Could you check a few things on this drawing? It's one solid part, dimensions in mm from its lowest x, y, z. A direction names the side the tool comes from. Give positions to 0.01 mm unless a question says otherwise; leave off trailing zeros. Loops run counter-clockwise (first coordinate to the right, second up) from the corner with the lowest first, then second, coordinate; pieces in that order, holes last. Notation, with made-up numbers: (85.25, 39.5) - (111.25, 39.5) arc R29 ccw to (111.25, 60.5) - close; hole circle Ø2 at (54, -22.75). An arc over 180 degrees is marked (long way). Return JSON: item names as keys, results as strings. Group by question number.
(1) If we mould it in two halves opening along X, with no side actions, what happens to the marked faces 3, 4, 5 and 6? For each: released by +X, released by -X, zero draft, split by the parting line, or undercut.
(2) I need wall thicknesses on probe 1 along X at (y, z) = (2.95, 6.5); probe 2 along Y at (x, z) = (10.25, 7.25). Which ranges of each line are inside material? Lowest first, please. Write a range as [from, to].
(3) For P1, Ø4.5, axis at x = 6, z = 5.5, coming from the +Y side; P2, Ø1.5, axis at x = 2.5, y = 0.5, coming from the +Z side, each with a flat end and sliding along its axis, tell me the tip position at first contact or that it passes through.
(4) If we section it at B-B (y = 4.75): Please give me the cut outline in (x, z), then the cut area to 3 significant figures.
(5) On a 3-axis mill with a long thin cutter (end or side, diameter ignored), from which of +Z, -Z, +X, -X, +Y, -Y can I reach the whole of each face in a straight line? I mean the marked faces 1 and 2. Say none if no direction works.
(6) If we section it at A-A (z = 6.5): Please give me the cut outline in (x, y).
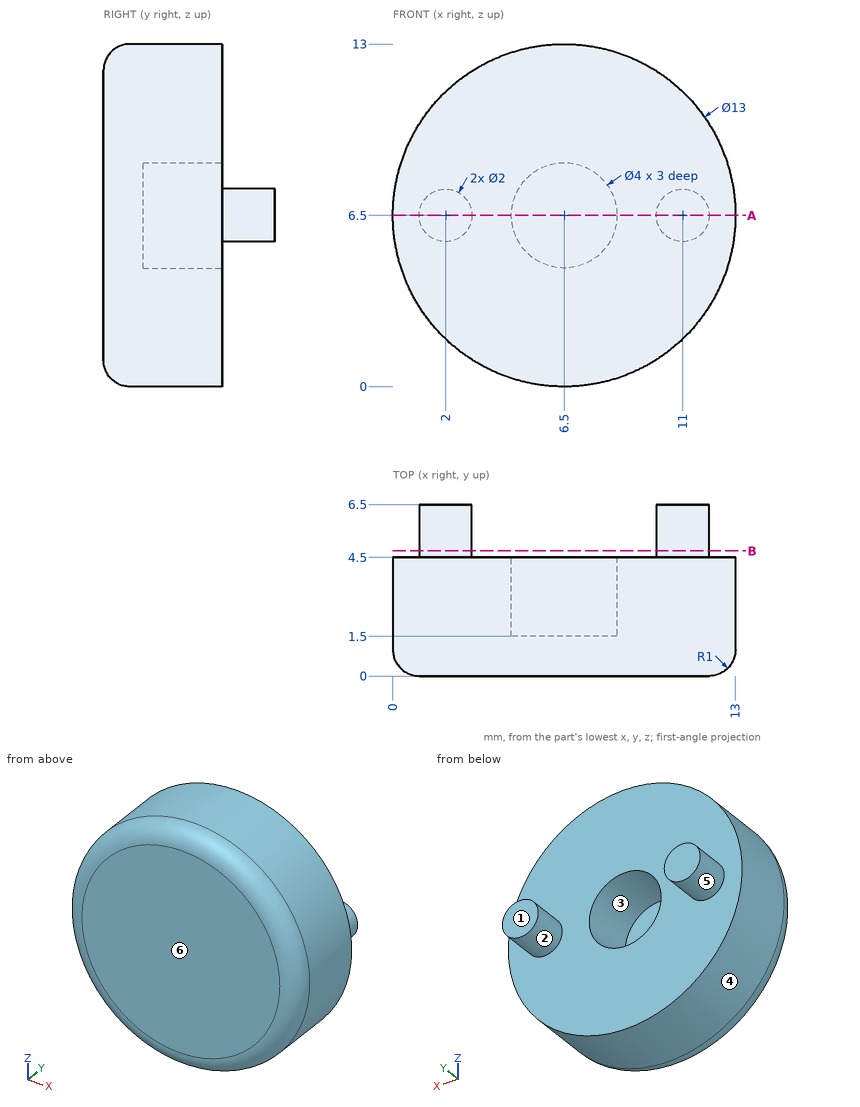
Values:
{
 "1": {"face 3": "undercut", "face 4": "split by the parting line", "face 5": "undercut", "face 6": "zero draft"},
 "2": {"probe 1": "[0, 4.5], [8.5, 13]", "probe 2": "[0, 4.5]"},
 "3": {"P1": "y = 4.5", "P2": "z = 12.07"},
 "4": {"outline": "circle Ø2 at (2, 6.5); circle Ø2 at (11, 6.5)", "area": "6.28 mm2"},
 "5": {"face 1": "+Z, -Z, +X, -X, +Y", "face 2": "+Y"},
 "6": {"outline": "(0, 1) arc R1 ccw to (1, 0) - (12, 0) arc R1 ccw to (13, 1) - (13, 4.5) - (12, 4.5) - (12, 6.5) - (10, 6.5) - (10, 4.5) - (8.5, 4.5) - (8.5, 1.5) - (4.5, 1.5) - (4.5, 4.5) - (3, 4.5) - (3, 6.5) - (1, 6.5) - (1, 4.5) - (0, 4.5) - close"}
}
